from build123d import *

# Parameters (mm, degrees)
F0_W     = 20
F0_H     = 25
F1_DEPTH = 50
F2_R     = 10
F3_R     = 2


with BuildPart() as f1:
    # F0 (on Right) → F1 (new body)
    with BuildSketch(Plane.YZ):
        Polygon((65.694234, 15), (-34.305766, 15), (-34.305766, 0), (-14.305766, 0), (45.694234, 0), (65.694234, 0), align=None)
        with Locations((-24.305766, -12.5)):
            Rectangle(F0_W, F0_H)
        with Locations((55.694234, -12.5)):
            Rectangle(F0_W, F0_H)
    extrude(amount=F1_DEPTH)

    # F2
    f2_edges = [f1.edges().sort_by_distance(p)[0] for p in [
        (25, -34.305766, 15),
        (25, 65.694234, 15),
    ]]
    fillet(f2_edges, radius=F2_R)

    # F3
    f3_edges = [f1.edges().sort_by_distance(p)[0] for p in [
        (50, 15.694234, 15),
        (0, 15.694234, 15),
    ]]
    fillet(f3_edges, radius=F3_R)


solid = f1.part
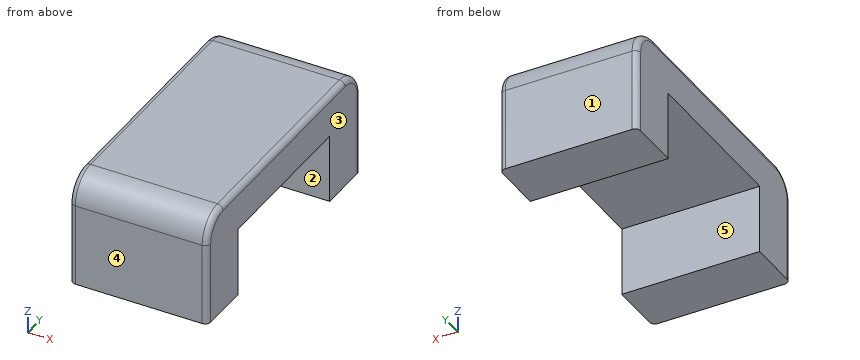
Could you check a few things on this model? Use its own coordinates, in mm. Face numbers are marked on the shaded views. A direction names the side the tool comes from. Coordinates: 2 decimals unless noted, no trailing zeros. Write each loop counter-clockwise with the first axis right and the second up, starting at its lowest first coordinate (ties: lowest second). Pieces come first, ordered by that corner, then holes. Notation, with made-up numbers: (36, -7.75) - (83, -7.75) arc R16 cw to (83, 3.25) - close; hole circle Ø6 at (-14.5, 61). An arc over 180 degrees is marked (long way). Put each result on its own line as item: value. Start each with the question number.
Q1. Which directions (+Z, -Z, +X, -X, +Y, -Y) give clear straight access to the entire face, cutting with the end or side of a thin tool? Please do the marked faces 1 and 2.
Q2. I want a section at C-C on y = -12. Write out the boundary of the cut face in (x, z).
Q3. Thinking about a two-plate mould opening in Y: for the marked faces 3, 4 and 5, which applies, pulls with the +Y half, pulls with the -Y half, needs draft (parallel to the pull), parting line crosses it, or undercut?
Q4. Please list where these lines run through material, in increasing order: L1, parallel to Y at x = 23, z = -6; L2, parallel to Z at x = 14, y = 35; L3, parallel to Z at x = 26.5, y = -24.5.
Q5. I want a section at A-A on z = -21. Write out the boundary of the cut face in (x, y).
Q6. I want a section at B-B on x = 33. Write out the boundary of the cut face in (y, z).
Q7. I'm going to push a flat-ended pin straight in: P1, Ø10, axis at x = 7.5, y = 16.5, coming from the -Z side. Where does the tip first touch, or does it pass through?
Checks:
1. face 1: +Z, -Z, +X, -X, +Y
1. face 2: -Z, +X, -X
2. outline: (0, 0) - (50, 0) - (50, 13) arc R2 ccw to (48, 15) - (2, 15) arc R2 ccw to (0, 13) - close
3. face 3: needs draft
3. face 4: pulls with the -Y half
3. face 5: undercut
4. L1: -34.31 to -14.31, 45.69 to 65.69
4. L2: 0 to 15
4. L3: -25 to 15
5. outline: (0, -32.31) arc R2 ccw to (2, -34.31) - (48, -34.31) arc R2 ccw to (50, -32.31) - (50, -14.31) - (0, -14.31) - close; (0, 45.69) - (50, 45.69) - (50, 63.69) arc R2 ccw to (48, 65.69) - (2, 65.69) arc R2 ccw to (0, 63.69) - close
6. outline: (-34.31, -25) - (-14.31, -25) - (-14.31, 0) - (45.69, 0) - (45.69, -25) - (65.69, -25) - (65.69, 5) arc R10 ccw to (55.69, 15) - (-24.31, 15) arc R10 ccw to (-34.31, 5) - close
7. P1: z = 0
